Here's how the part is built. I have some questions about the finished solid (model axes, mm). Face numbers are marked on the shaded views. Coordinates: 2 decimals unless noted, no trailing zeros. Write each loop counter-clockwise with the first axis right and the second up, starting at its lowest first coordinate (ties: lowest second). Pieces come first, ordered by that corner, then holes. Notation, with made-up numbers: M 53.5,84 L 107.5,84 A25 ccw 107.5,106 Z; hole C 10,-40 d8. An arc over 180 degrees is marked long. Use a Markdown table: item, result.
```python
from build123d import *

# Parameters (mm, degrees)
F0_W     = 120
F0_H     = 120
F0_R     = 2.05
F1_DEPTH = 5
F2_W     = 120
F2_H     = 120
F2_W_2   = 110
F2_H_2   = 110
F3_DEPTH = 5


with BuildPart() as f1:
    # F0 (on Top) → F1 (new body)
    with BuildSketch(Plane.XY):
        Rectangle(F0_W, F0_H)
        with Locations((-13, -50)):
            Circle(F0_R, mode=Mode.SUBTRACT)
        with Locations((-13, -17.5)):
            Circle(F0_R, mode=Mode.SUBTRACT)
        with Locations((13, -50)):
            Circle(F0_R, mode=Mode.SUBTRACT)
        with Locations((13, -17.5)):
            Circle(F0_R, mode=Mode.SUBTRACT)
        with Locations((-13, 17.5)):
            Circle(F0_R, mode=Mode.SUBTRACT)
        with Locations((-13, 50)):
            Circle(F0_R, mode=Mode.SUBTRACT)
        with Locations((13, 17.5)):
            Circle(F0_R, mode=Mode.SUBTRACT)
        with Locations((13, 50)):
            Circle(F0_R, mode=Mode.SUBTRACT)
    extrude(amount=-F1_DEPTH)

    # F2 (on Top) → F3 (join)
    with BuildSketch(Plane.XY):
        Rectangle(F2_W, F2_H)
        Rectangle(F2_W_2, F2_H_2, mode=Mode.SUBTRACT)
    extrude(amount=F3_DEPTH)


solid = f1.part
```
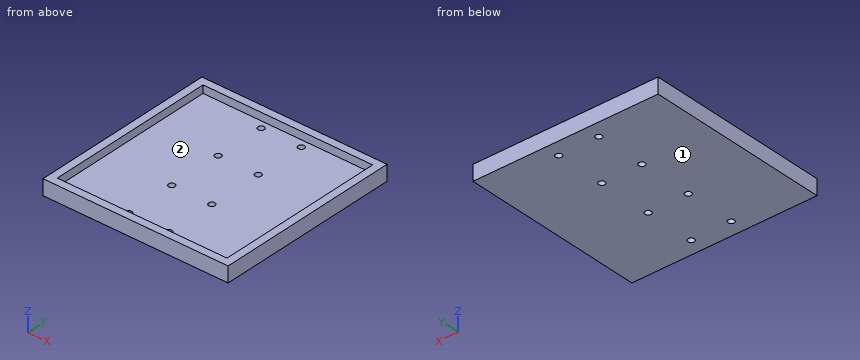
1. I need wall thicknesses on probe 1 along Y at (x, z) = (13, -3.9); probe 2 along X at (y, z) = (-49.5, 1.75). Which ranges of each line are inside material? Lowest first, please.
Answers follow:
| item | result |
|---|---|
| probe 1 | y = -60 to -52.05, -47.95 to -19.55, -15.45 to 15.45, 19.55 to 47.95, 52.05 to 60 |
| probe 2 | x = -60 to -55, 55 to 60 |
2. Will these pins go through, and if not, where does the flat tip stop? pin 1 Ø2.5 at (x, y) = (-13, -17.5) entering from -Z; pin 2 Ø6.5 at (x, y) = (-13, -50) entering from +Z.
Answers follow:
| item | result |
|---|---|
| pin 1 | passes through |
| pin 2 | stops at z = 0 |
3. We'd pull the mould along Y, two halves only. Please class the marked faces 1 and 2: +Y half, -Y half, draft (parallel to the pull), parting line (faces both ways), or undercut.
Answers follow:
| item | result |
|---|---|
| face 1 | draft |
| face 2 | undercut |
4. Suppose I cut it at B-B on y = 50. Write out the boundary of the cut face in (x, z).
Answers follow:
| item | result |
|---|---|
| outline | M -60,-5 L -15.05,-5 L -15.05,0 L -55,0 L -55,5 L -60,5 Z; M -10.95,-5 L 10.95,-5 L 10.95,0 L -10.95,0 Z; M 15.05,-5 L 60,-5 L 60,5 L 55,5 L 55,0 L 15.05,0 Z |
5. Suppose I cut it at A-A on x = 13. Write out the boundary of the cut face in (y, z).
Answers follow:
| item | result |
|---|---|
| outline | M -60,-5 L -52.05,-5 L -52.05,0 L -55,0 L -55,5 L -60,5 Z; M -47.95,-5 L -19.55,-5 L -19.55,0 L -47.95,0 Z; M -15.45,-5 L 15.45,-5 L 15.45,0 L -15.45,0 Z; M 19.55,-5 L 47.95,-5 L 47.95,0 L 19.55,0 Z; M 52.05,-5 L 60,-5 L 60,5 L 55,5 L 55,0 L 52.05,0 Z |
6. Suppose I cut it at C-C on x = -18.5. Write out the boundary of the cut face in (y, z), and give its area (3 significant figures).
Answers follow:
| item | result |
|---|---|
| outline | M -60,-5 L 60,-5 L 60,5 L 55,5 L 55,0 L -55,0 L -55,5 L -60,5 Z |
| area | 650 mm2 |
